from build123d import *

# Parameters (mm, degrees)
SKETCH1_R           = 88.9
SKETCH1_R_2         = 76.2
BOSS_EXTRUDE1_DEPTH = 7.9375
SKETCH2_R           = 88.9
SKETCH2_R_2         = 69.85
BOSS_EXTRUDE2_DEPTH = 3.175
SKETCH3_R           = 2.5
CUT_EXTRUDE1_DEPTH  = 127.213737985
CIRPATTERN1_COUNT   = 6


with BuildPart() as part:
    # Sketch1 → Boss-Extrude1 (new body)
    with BuildSketch(Plane(origin=(0, 0, 0), x_dir=(1, 0, 0), z_dir=(0, 1, 0))):
        with Locations(Location((0, 0, 0), (0, 0, 270))):
            Circle(SKETCH1_R)
        with Locations(Location((0, 0, 0), (0, 0, 270))):
            Circle(SKETCH1_R_2, mode=Mode.SUBTRACT)
    extrude(amount=BOSS_EXTRUDE1_DEPTH)

    # Sketch2 → Boss-Extrude2 (add)
    with BuildSketch(Plane(origin=(0, 7.9375, 0), x_dir=(1, 0, 0), z_dir=(0, 1, 0))):
        with Locations(Location((0, 0, 0), (0, 0, 270))):
            Circle(SKETCH2_R)
        with Locations(Location((0, 0, 0), (0, 0, 270))):
            Circle(SKETCH2_R_2, mode=Mode.SUBTRACT)
    extrude(amount=BOSS_EXTRUDE2_DEPTH)

    # Sketch3 → Cut-Extrude1 (cut, through all)
    with BuildSketch(Plane(origin=(0, 11.1125, 0), x_dir=(1, 0, 0), z_dir=(0, 1, 0))):
        with Locations(Location((0, 82.55, 0), (0, 0, 270))):
            Circle(SKETCH3_R)
    cut_extrude1 = extrude(amount=-CUT_EXTRUDE1_DEPTH, mode=Mode.SUBTRACT)

    # CirPattern1: Cut-Extrude1 ×6 about axis
    cirpattern1_axis = Axis((0, 0, 0), (0, 1, 0))
    for i in range(1, CIRPATTERN1_COUNT):
        add(cut_extrude1.rotate(cirpattern1_axis, i * 360 / CIRPATTERN1_COUNT), mode=Mode.SUBTRACT)


solid = part.part
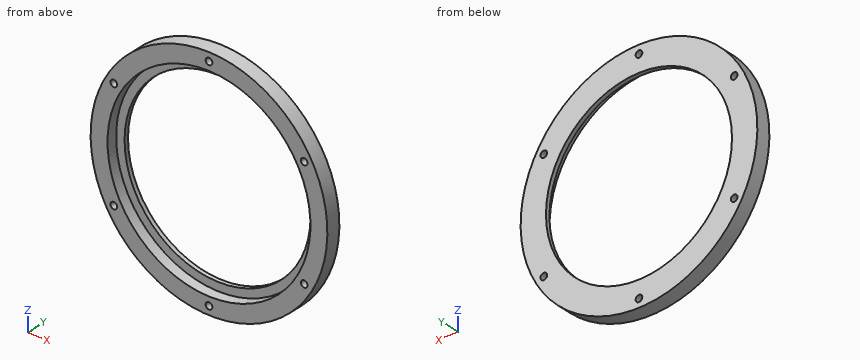
Can you work these out from the model? Positions are in its coordinate system, mm. Give positions to 0.01 mm unless a question says otherwise; leave off trailing zeros. Order: outer loops, then holes, each group sorted by start corner. A loop starts at its lowest first (then second) coordinate and runs counter-clockwise, first axis right, second up. Notation, with made-up numbers: M 12.5,-8 L 63.5,-8 A27 cw 63.5,28 Z; hole C 84.25,-5.5 d10. An arc over 180 degrees is marked long. Use a Markdown table: item, result. Add a question column.
Item 1: Suppose I cut it at D-D (x = -46). List the corners of the cut face in (y, z) for me.
Item 2: Suppose I cut it at C-C (y = 4.5). List the corners of the cut face in (x, z) for me (3 decimals).
Item 3: If I drill on L1, parallel to X at y = 9.2, z = 0; L2, parallel to Y at x = 44, z = 61; L3, parallel to Z at x = -30.5, y = 2.5, over which ranges is the centre line in solid material (lowest first)? Write a range as [from, to].
Item 4: Suppose I cut it at A-A (x = 0). List the corners of the cut face in (y, z) for me, then the cut area to 3 significant figures.
Item 5: Suppose I cut it at B-B (z = 0). List the corners of the cut face in (x, y) for me.
Item 6: Will these pins go through, and if not, where does the flat tip stop? pin 1 (3 mm diameter, centred on x = 71.49, z = 41.28, fed in from +Y); pin 2 (1.5 mm diameter, centred on x = -20, y = 2, fed in from +Z); pin 3 (6 mm diameter, centred on y = 7, z = 7, fed in from +X); pin 4 (3 mm diameter, centred on y = 7.5, z = -54.5, fed in from -X).
Answer sheet:
| question | item | result |
|---|---|---|
| 1 | outline | M 0,-76.07 L 11.11,-76.07 L 11.11,-52.56 L 7.94,-52.56 L 7.94,-60.75 L 0,-60.75 Z; M 0,60.75 L 7.94,60.75 L 7.94,52.56 L 11.11,52.56 L 11.11,76.07 L 0,76.07 Z |
| 2 | outline | C 0,0 d177.8; hole C 0,0 d152.4; hole C -71.49,-41.275 d5; hole C -71.49,41.275 d5; hole C 0,-82.55 d5; hole C 0,82.55 d5; hole C 71.49,-41.275 d5; hole C 71.49,41.275 d5 |
| 3 | L1 | x = [-88.9, -69.85], [69.85, 88.9] |
| 3 | L2 | y = [7.94, 11.11] |
| 3 | L3 | z = [-83.5, -69.83], [69.83, 83.5] |
| 4 | outline | M 0,-88.9 L 11.11,-88.9 L 11.11,-85.05 L 0,-85.05 Z; M 0,-80.05 L 11.11,-80.05 L 11.11,-69.85 L 7.94,-69.85 L 7.94,-76.2 L 0,-76.2 Z; M 0,76.2 L 7.94,76.2 L 7.94,69.85 L 11.11,69.85 L 11.11,80.05 L 0,80.05 Z; M 0,85.05 L 11.11,85.05 L 11.11,88.9 L 0,88.9 Z |
| 4 | area | 211 mm² |
| 5 | outline | M -88.9,0 L -76.2,0 L -76.2,7.94 L -69.85,7.94 L -69.85,11.11 L -88.9,11.11 Z; M 69.85,7.94 L 76.2,7.94 L 76.2,0 L 88.9,0 L 88.9,11.11 L 69.85,11.11 Z |
| 6 | pin 1 | passes through |
| 6 | pin 2 | stops at z = 86.79 |
| 6 | pin 3 | stops at x = 88.81 |
| 6 | pin 4 | stops at x = -71.37 |
